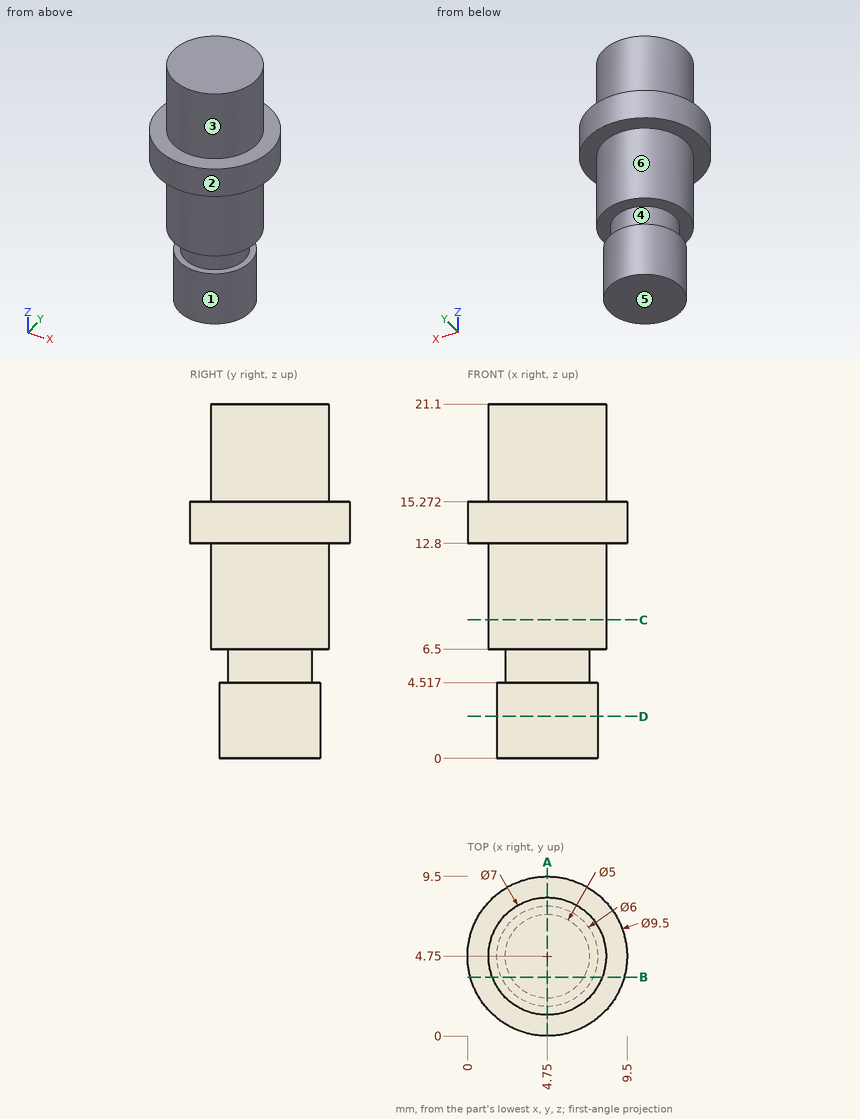
The drawing under review shows one solid part. Ordinate dimensions are in mm from its lowest x, y, z. A direction names the side the tool comes from. Give positions to 0.01 mm unless a question says otherwise; leave off trailing zeros. Loops run counter-clockwise (first coordinate to the right, second up) from the corner with the lowest first, then second, coordinate; pieces in that order, holes last. Notation, with made-up numbers: M -34,6.25 L 9,6.25 A8 cw 9,19.25 Z; hole C 14.5,12.5 d5. An arc over 180 degrees is marked long. One line per question, with ' | ' between items. Start each with the question number.
1. Add section D-D (z = 2.5). Write out the cut boundary in (x, y).
2. Add section A-A (x = 4.75). Write out the cut boundary in (y, z), plus the area to 3 significant figures.
3. For the marked faces 1, 2 and 3, list the 3-axis set-ups (+Z, -Z, +X, -X, +Y, -Y) from which the entire face can be reached by the end or side of a thin tool; tool diameter is ignored.
4. To check wall thickness, follow L1, parallel to Z at x = 2, y = 4.75; L2, parallel to Z at x = 1.5, y = 2; L3, parallel to Z at x = 1.5, y = 4.25. State the ranges of each line that lie inside material, in increasing order.
5. The part is to be moulded in two halves that separate along Z. For the marked faces 4, 5 and 6, say which applies: released by +Z, released by -Z, zero draft, split by the parting line, or undercut.
6. Insertion check: P1, Ø1.5, axis at x = 2.5, z = 8, coming from the +Y side; P2, Ø3, axis at y = 5.5, z = 10, coming from the -X side; P3, Ø5, axis at y = 3, z = 6, coming from the +X side. Each pin has a flat end and moves straight along its axis. Give the tip position at first contact, or say it passes through.
7. Add section B-B (y = 3.5). Write out the cut boundary in (x, z) (1 decimal), plus the area to 3 significant figures.
8. Add section C-C (z = 8.25). Write out the cut boundary in (x, y).
Worked out:
1) outline: C 4.75,4.75 d6
2) outline: M 0,12.8 L 1.25,12.8 L 1.25,6.5 L 2.25,6.5 L 2.25,4.52 L 1.75,4.52 L 1.75,0 L 7.75,0 L 7.75,4.52 L 7.25,4.52 L 7.25,6.5 L 8.25,6.5 L 8.25,12.8 L 9.5,12.8 L 9.5,15.27 L 8.25,15.27 L 8.25,21.1 L 1.25,21.1 L 1.25,15.27 L 0,15.27 Z | area: 145 mm²
3) face 1: -Z | face 2: +Z, -Z | face 3: +Z
4) L1: z = 0 to 4.52, 6.5 to 21.1 | L2: z = 12.8 to 15.27 | L3: z = 6.5 to 21.1
5) face 4: undercut | face 5: released by -Z | face 6: zero draft
6) P1: stops at y = 7.91 | P2: stops at x = 1.25 | P3: stops at x = 8.25
7) outline: M 0.2,12.8 L 1.5,12.8 L 1.5,6.5 L 2.6,6.5 L 2.6,4.5 L 2,4.5 L 2,0 L 7.5,0 L 7.5,4.5 L 6.9,4.5 L 6.9,6.5 L 8,6.5 L 8,12.8 L 9.3,12.8 L 9.3,15.3 L 8,15.3 L 8,21.1 L 1.5,21.1 L 1.5,15.3 L 0.2,15.3 Z | area: 135 mm²
8) outline: C 4.75,4.75 d7
